The model under review builds one solid part; all positions refer to its coordinate system, in mm. Face numbers are marked on the shaded views. A direction names the side the tool comes from. Round coordinates to 2 decimals unless told otherwise and drop trailing zeros. Loops run counter-clockwise (first coordinate to the right, second up) from the corner with the lowest first, then second, coordinate; pieces in that order, holes last. Notation, with made-up numbers: (2.25, 3) -> (35.25, 3) arc R15 cw to (35.25, 11) -> close; hole circle Ø6 at (35.25, -18). An arc over 180 degrees is marked (long way). Write each question's results on one line, items separated by ' | '. Start each with the question number.
Item 1: We need section B-B (y = 15). Give the boundary of the cut face in (x, z).
Item 2: Mouldability with a two-part tool opening along X and no side actions: class the marked faces 4, 5, 6 and 7 as pulls with the +X half, pulls with the -X half, needs draft (parallel to the pull), parting line crosses it, or undercut.
Item 3: Tool access review of the marked faces 1, 2 and 3: name each direction out of +Z, -Z, +X, -X, +Y, -Y from which nothing blocks a thin tool from reaching the whole face with its end or side.
Item 4: Clearance check with flat-ended pins moving along their axes: pin 1 Ø9.5 at (y, z) = (22, -21) entering from +X; pin 2 Ø12 at (x, z) = (30, -10.5) entering from +Y; pin 3 Ø5.5 at (x, z) = (51, -21) entering from +Y. State where each tip first meets the part, or that it passes through.
Item 5: We need section A-A (x = 17). Give the boundary of the cut face in (y, z), and give its area (3 significant figures).
Item 6: We need section D-D (y = 22). Give the boundary of the cut face in (x, z).
Item 7: We need section C-C (z = -2.25). Give the boundary of the cut face in (x, y), and give its area (3 significant figures).
Item 8: For L1, parallel to Z at x = 1.15, y = 22; L2, parallel to Z at x = 1.95, y = 22; L3, parallel to Y at x = 1.9, z = -21, list the stretches that pass through material, from the lowest coordinate up. Write a range as from..to.
Autodesk Inventor part; units mm, degrees
ref_plane "YZ Plane" through (0, 0, 0) normal (1, 0, 0) x (0, 1, 0)
ref_plane "XZ Plane" through (0, 0, 0) normal (0, 1, 0) x (-1, 0, 0)
ref_plane "XY Plane" through (0, 0, 0) normal (0, 0, 1) x (1, 0, 0)
sketch "Skizze1" plane through (0, 0, 0) normal (0, 0, 1) x (1, 0, 0)
  line L0 (0, 0) -> (55, 0)
  line L1 (55, 0) -> (55, 26)
  line L2 (55, 26) -> (0, 26)
  line L3 (0, 26) -> (0, 0)
  circle A0 centre (17, 15) radius 8.75
  circle A1 centre (42.5, 15) radius 8.75
  dimension "D" = 17.5
  dimension "d1" = 17.5
  dimension "Hoehe" = 26
  dimension "L" = 55
  dimension "d5" = 17
  dimension "d7" = 11
  dimension "d14" = 12.5
extrude "Extrusion1" add sketch "Skizze1" along normal blind 3
sketch "Skizze2" plane through (0, 0, 0) normal (0, 0, -1) x (-1, 0, 0)
  line L0 (-55, 0) -> (-55, 26)
  line L1 (0, 0) -> (-55, 0)
  line L2 (0, 26) -> (0, 0)
  line L3 (-55, 26) -> (0, 26)
  circle A0 centre (-17, 15) radius 8.75
  circle A1 centre (-42.5, 15) radius 8.75
  line L4 (-55, 26) -> (0, 26)
  line L5 (-3, 26) -> (-3, 3)
  line L6 (-3, 3) -> (-55, 3)
  dimension "Dicke" = 3
  dimension "d11" = 3
extrude "Extrusion2" add sketch "Skizze2" along normal blind 25 contours L0 L6 L5 L3 L2 L1
sketch "Skizze3" plane through (3, 3, 0) normal (0, 1, 0) x (1, 0, 0)
  line L0 (52, 0) -> (52, 25)
  line L1 (0, 25) -> (52, 25)
  point P0 (-3, 0)
  point P1 (48, 21)
  dimension "d22" = 4
  dimension "d23" = 4
hole "Bohrung1" at (51, 3, -21) direction (0, -1, 0) diameter 3.5 end through all counterbore diameter 6 counterbore depth 1.5
sketch "Skizze4" plane through (3, 3, 0) normal (1, 0, 0) x (0, 0, -1)
  line L0 (0, 23) -> (25, 23)
  line L1 (25, 23) -> (25, 0)
  point P0 (0, -3)
  point P1 (21, 19)
  dimension "d31" = 4
  dimension "d32" = 4
hole "Bohrung2" at (3, 22, -21) direction (-1, 0, 0) diameter 3.5 end through all counterbore diameter 6 counterbore depth 1.5
sketch "Skizze5" plane through (0, 0, -25) normal (0, 0, -1) x (-1, 0, 0)
  circle A0 centre (-42.5, 15) radius 8.75
  circle A1 centre (-17, 15) radius 8.75
  circle A2 centre (-42.5, 15) radius 14
  circle A3 centre (-17, 15) radius 14
  point P0 (0, 0)
  point P1 (-29.75, 9.2175)
  point P2 (-29.75, 20.7825)
  dimension "d33" = 28
  dimension "d34" = 28
extrude "Extrusion3" cut sketch "Skizze5" against normal blind 25 contours A2 A3 | A3 A2 picked at (-4.9763, 13.1615) picked at (-54.5237, 16.8385)
equation "\"d1\" = D"
equation "\"d11\" = Dicke"
equation "\"d34\" = d33"
properties part number "Buttons_Mount_v2"
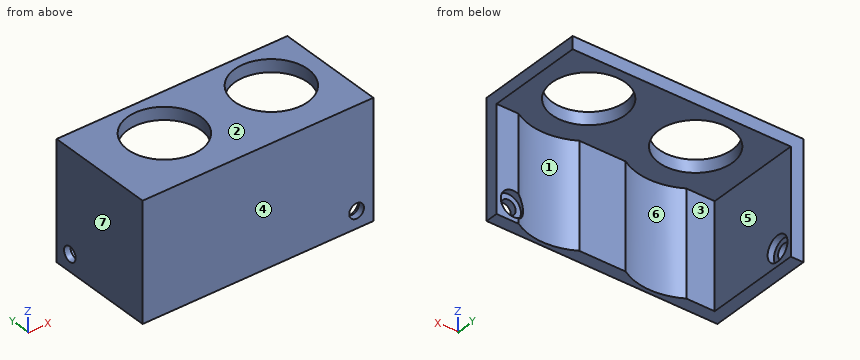
Here are the results:
1) outline: (0, -25) -> (3, -25) -> (3, 0) -> (8.25, 0) -> (8.25, 3) -> (0, 3) -> close; (25.75, 0) -> (33.75, 0) -> (33.75, 3) -> (25.75, 3) -> close; (51.25, 0) -> (55, 0) -> (55, 3) -> (51.25, 3) -> close
2) face 4: needs draft | face 5: pulls with the +X half | face 6: undercut | face 7: pulls with the -X half
3) face 1: -Z, +Y | face 2: +Z, +X, -X, +Y, -Y | face 3: -Z, +X, +Y
4) pin 1: stops at x = 3 | pin 2: stops at y = 3 | pin 3: stops at y = 1.5
5) outline: (0, -25) -> (1, -25) -> (1, 0) -> (6.25, 0) -> (6.25, 3) -> (0, 3) -> close; (23.75, 0) -> (26, 0) -> (26, 3) -> (23.75, 3) -> close | area: 50.5 mm2
6) outline: (0, -25) -> (3, -25) -> (3, -24) -> (1.5, -24) -> (1.5, -22.75) -> (0, -22.75) -> close; (0, -19.25) -> (1.5, -19.25) -> (1.5, -18) -> (3, -18) -> (3, 0) -> (11.75, 0) -> (11.75, 3) -> (0, 3) -> close; (22.25, 0) -> (37.25, 0) -> (37.25, 3) -> (22.25, 3) -> close; (47.75, 0) -> (55, 0) -> (55, 3) -> (47.75, 3) -> close
7) outline: (0, 0) -> (55, 0) -> (55, 3) -> (49.71, 3) arc R14 cw to (35.29, 3) -> (24.21, 3) arc R14 cw to (9.79, 3) -> (3, 3) -> (3, 26) -> (0, 26) -> close | area: 195 mm2
8) L1: z = -25..-22.75, -19.25..3 | L2: z = -25..-24, -18..3 | L3: y = 0..19, 25..26
